from build123d import *

# Parameters (mm, degrees)
SKETCH_1_W          = 25
SKETCH_1_H          = 80
SKETCH_1_W_2        = 30
EXTRUDE_1_DEPTH     = 30
SKETCH_2_W          = 40
SKETCH_2_H          = 80
EXTRUDE_2_DEPTH     = 80
FILLET_1_R          = 40
SKETCH_3_R          = 7.5
CUT_EXTRUDE_1_DEPTH = 142.774468788
SKETCH_6_W          = 170
SKETCH_6_H          = 150
EXTRUDE_5_DEPTH     = 20
SKETCH_7_W          = 170
SKETCH_7_H          = 20
EXTRUDE_6_DEPTH     = 150
EXTRUDE_7_DEPTH     = 40
SKETCH_10_R         = 2
CUT_EXTRUDE_3_DEPTH = 241.312296814
SKETCH_11_W         = 50
SKETCH_11_H         = 80
EXTRUDE_8_DEPTH     = 110
SKETCH_12_W         = 80
SKETCH_12_H         = 40
CUT_EXTRUDE_4_DEPTH = 267.505159425
SKETCH_13_R         = 12.5
CUT_EXTRUDE_5_DEPTH = 259.89186932
SKETCH_14_R         = 5
CUT_EXTRUDE_6_DEPTH = 259.89186932
SKETCH_15_W         = 21.752867029
SKETCH_15_H         = 110
EXTRUDE_9_DEPTH     = 50
SKETCH_16_R         = 2
CUT_EXTRUDE_7_DEPTH = 21.752867029
SKETCH_17_R         = 2
CUT_EXTRUDE_8_DEPTH = 20


with BuildPart() as part:
    # Sketch 1 → Extrude 1 (new body)
    with BuildSketch(Plane.XY):
        with Locations((12.5, -40)):
            Rectangle(SKETCH_1_W, SKETCH_1_H)
        with Locations((40, -40)):
            Rectangle(SKETCH_1_W_2, SKETCH_1_H)
        with Locations((67.5, -40)):
            Rectangle(SKETCH_1_W, SKETCH_1_H)
    extrude(amount=EXTRUDE_1_DEPTH)

    # Sketch 2 → Extrude 2 (add)
    with BuildSketch(Plane.XY.offset(30)):
        with Locations((60, -40)):
            Rectangle(SKETCH_2_W, SKETCH_2_H)
    extrude(amount=EXTRUDE_2_DEPTH)

    # Fillet 1
    fillet_1_edges = [part.edges().sort_by_distance(p)[0] for p in [
        (60, 0, 110),
        (60, -80, 110),
    ]]
    fillet(fillet_1_edges, radius=FILLET_1_R - 0.0001)  # a hair under: the kernel refuses the full size

    # Sketch 3 → Cut-Extrude 1 (cut, through all)
    with BuildSketch(Plane.ZY.offset(-40)):
        with Locations(Location((70, -40, 0), (0, 0, 270))):
            Circle(SKETCH_3_R)
    extrude(amount=-CUT_EXTRUDE_1_DEPTH, mode=Mode.SUBTRACT)



with BuildPart() as body_2:
    # Sketch 6 → Extrude 5 (new body)
    with BuildSketch(Plane(origin=(0, 0, 0), x_dir=(-1, 0, 0), z_dir=(0, 0, -1))):
        with Locations((-40, -40)):
            Rectangle(SKETCH_6_W, SKETCH_6_H)
    extrude(amount=EXTRUDE_5_DEPTH)

    # Sketch 7 → Extrude 6 (add)
    with BuildSketch(Plane(origin=(0, 0, -20), x_dir=(-1, 0, 0), z_dir=(0, 0, -1))):
        with Locations((-40, 25)):
            Rectangle(SKETCH_7_W, SKETCH_7_H)
        with Locations((-40, -105)):
            Rectangle(SKETCH_7_W, SKETCH_7_H)
    extrude(amount=EXTRUDE_6_DEPTH)


with BuildPart() as part_1:
    add(part.part)

    add(body_2.part)  # Extrude 7 merges body 2
    # Sketch 9 → Extrude 7 (add)
    with BuildSketch(Plane(origin=(80, 0, 0), x_dir=(0, 0, -1), z_dir=(1, 0, 0))):
        with BuildLine():
            ThreePointArc((-70, -80), (-78.559038333, -79.073557079), (-86.721603642, -76.337143141))
            Line((-86.721603642, -76.337143141), (-86.721603642, -91.337143141))
            Line((-86.721603642, -91.337143141), (0, -91.337143141))
            Line((0, -91.337143141), (0, -80))
            Line((0, -80), (-70, -80))
        make_face()
    extrude(amount=-EXTRUDE_7_DEPTH)

    # Sketch 10 → Cut-Extrude 3 (cut, through all)
    with BuildSketch(Plane(origin=(80, 0, 0), x_dir=(0, 0, -1), z_dir=(1, 0, 0))):
        with Locations(Location((-70, -85, 0), (0, 0, 90))):
            Circle(SKETCH_10_R)
    extrude(amount=-CUT_EXTRUDE_3_DEPTH, mode=Mode.SUBTRACT)

    # Sketch 11 → Extrude 8 (add)
    with BuildSketch(Plane(origin=(0, -95, 0), x_dir=(1, 0, 0), z_dir=(0, 1, 0))):
        with Locations((-20, 130)):
            Rectangle(SKETCH_11_W, SKETCH_11_H)
        with Locations((100, 130)):
            Rectangle(SKETCH_11_W, SKETCH_11_H)
    extrude(amount=EXTRUDE_8_DEPTH)

    # Sketch 12 → Cut-Extrude 4 (cut, through all)
    with BuildSketch(Plane(origin=(125, 0, 0), x_dir=(0, 0, -1), z_dir=(1, 0, 0))):
        with Locations((130, -40)):
            Rectangle(SKETCH_12_W, SKETCH_12_H)
    extrude(amount=-CUT_EXTRUDE_4_DEPTH, mode=Mode.SUBTRACT)

    # Sketch 13 → Cut-Extrude 5 (cut, through all)
    with BuildSketch(Plane(origin=(0, 35, 0), x_dir=(1, 0, 0), z_dir=(0, 1, 0))):
        with Locations(Location((100, 130, 0), (0, 0, 180))):
            Circle(SKETCH_13_R)
        with Locations(Location((-20, 130, 0), (0, 0, 180))):
            Circle(SKETCH_13_R)
    extrude(amount=-CUT_EXTRUDE_5_DEPTH, mode=Mode.SUBTRACT)

    # Sketch 14 → Cut-Extrude 6 (cut, through all)
    with BuildSketch(Plane.XZ.offset(115)):
        with Locations((0, -42.5)):
            Circle(SKETCH_14_R)
        with Locations(Location((80, -42.5, 0), (0, 0, 90))):
            Circle(SKETCH_14_R)
    extrude(amount=-CUT_EXTRUDE_6_DEPTH, mode=Mode.SUBTRACT)

    # Sketch 15 → Extrude 9 (add)
    with BuildSketch(Plane(origin=(0, 0, -20), x_dir=(-1, 0, 0), z_dir=(0, 0, -1))):
        with Locations((34.123566485, -40)):
            Rectangle(SKETCH_15_W, SKETCH_15_H)
    extrude(amount=EXTRUDE_9_DEPTH)

    # Sketch 16 → Cut-Extrude 7 (cut)
    with BuildSketch(Plane.ZY.offset(45)):
        with Locations(Location((-20, -80, 0), (0, 0, 270))):
            Circle(SKETCH_16_R)
        with Locations(Location((-40, -80, 0), (0, 0, 270))):
            Circle(SKETCH_16_R)
    extrude(amount=-CUT_EXTRUDE_7_DEPTH, mode=Mode.SUBTRACT)

    # Sketch 17 → Cut-Extrude 8 (cut)
    with BuildSketch(Plane.XZ.offset(115)):
        with Locations((-25, -110)):
            Circle(SKETCH_17_R)
        with Locations((25, -110)):
            Circle(SKETCH_17_R)
    extrude(amount=-CUT_EXTRUDE_8_DEPTH, mode=Mode.SUBTRACT)


solid = part_1.part
Could you check a few things on this model? Use its own coordinates, in mm. A direction names the side the tool comes from. Give positions to 0.01 mm unless a question says otherwise; leave off trailing zeros. Order: outer loops, then holes, each group sorted by start corner. A loop starts at its lowest first (then second) coordinate and runs counter-clockwise, first axis right, second up. Notation, with made-up numbers: (61, 12) -> (87, 12) arc R11 ccw to (87, 20) -> close; hole circle Ø5 at (-16, 38). An arc over 180 degrees is marked (long way). Answer in a Markdown table with one row per item. Add a question column.
Item 1: Please list where these lines run through material, in increasing order: probe 1 along Z at (x, y) = (-40, -80); probe 2 along Z at (x, y) = (53, -85); probe 3 along Y at (x, z) = (74.5, -83).
Item 2: Imagine slicing it at B-B (x = 100). List the corners of the cut face in (y, z) for me, and give its area (4 significant figures).
Item 3: We'd pull the mould along Z, two halves only. Please class faces 4 (the flat face through (80, -45, 56)), 5 (the flat face through (-34, -39, -70)), 6 (the flat face through (20, -39, 30)): pulls with the +Z half, pulls with the -Z half, needs draft (parallel to the pull), parting line crosses it, or undercut.
Item 4: Imagine slicing it at C-C (y = -17). List the corners of the cut face in (x, z) for me, and give its area (3 significant figures).
Item 5: Imagine slicing it at D-D (x = 69). Count the separate pieces of the cut face and the enclosed holes in it, and give its area (3 significant figures).
Item 6: For faces 1 (the flat face through (-20, -3, -90)), 2 (the flat face through (89, -60, -121)), 3 (the flat face through (75, -78, -129)), which set-ups out of +Z, -Z, +X, -X, +Y, -Y let a thin tool reach every point of the face, with its end or its side?
Item 7: I'm going to push flat-ended pins straight in: P1, Ø8, axis at x = 80, z = -42.5, coming from the +Y side; P2, Ø24, axis at x = 11, z = 14, coming from the -Y side; P3, Ø1, axis at y = -68, z = 44, coming from the -X side; P4, Ø4, axis at x = 11.5, y = -58, coming from the -Z side. Where does each tip first touch, or does it pass through?
Item 8: Imagine slicing it at A-A (z = -84). List the corners of the cut face in (x, y) for me.
Result:
| question | item | result |
|---|---|---|
| 1 | probe 1 | -170 to -90, -70 to -42, -38 to -22, -18 to 0 |
| 1 | probe 2 | -20 to 68, 72 to 86.72 |
| 1 | probe 3 | -115 to -95, 15 to 35 |
| 2 | outline | (-115, -170) -> (-60, -170) -> (-60, -142.5) -> (-115, -142.5) -> close; (-115, -117.5) -> (-60, -117.5) -> (-60, -90) -> (-95, -90) -> (-95, -20) -> (15, -20) -> (15, -90) -> (-20, -90) -> (-20, -117.5) -> (35, -117.5) -> (35, 0) -> (-115, 0) -> close; (-20, -170) -> (35, -170) -> (35, -142.5) -> (-20, -142.5) -> close |
| 2 | area | 11,850 mm2 |
| 3 | face 4 | needs draft |
| 3 | face 5 | undercut |
| 3 | face 6 | pulls with the +Z half |
| 4 | outline | (-45, -170) -> (5, -170) -> (5, -90) -> (-45, -90) -> close; (-45, -70) -> (-23.25, -70) -> (-23.25, -20) -> (125, -20) -> (125, 0) -> (80, 0) -> (80, 102.73) -> (40, 102.73) -> (40, 30) -> (0, 30) -> (0, 0) -> (-45, 0) -> close; (75, -170) -> (125, -170) -> (125, -90) -> (75, -90) -> close; hole circle Ø25 at (-20, -130); hole circle Ø25 at (100, -130) |
| 4 | area | 16,800 mm2 |
| 5 | separate pieces | 1 |
| 5 | enclosed holes | 2 |
| 5 | area | 17,900 mm2 |
| 6 | face 1 | +X, -X |
| 6 | face 2 | -Z, +X, -X |
| 6 | face 3 | -Z |
| 7 | P1 | through |
| 7 | P2 | y = -80 |
| 7 | P3 | x = 40 |
| 7 | P4 | z = -20 |
| 8 | outline | (-45, -115) -> (125, -115) -> (125, -95) -> (-45, -95) -> close; (-45, 15) -> (125, 15) -> (125, 35) -> (-45, 35) -> close |
